Part model, mm, in its own coordinate system. Face numbers are marked on the shaded views. A direction names the side the tool comes from. Give positions to 0.01 mm unless a question says otherwise; leave off trailing zeros. Write each loop counter-clockwise with the first axis right and the second up, starting at its lowest first coordinate (ties: lowest second). Pieces come first, ordered by that corner, then holes.
```python
from build123d import *

# Parameters (mm, degrees)
SKETCH1_R           = 10
BOSS_EXTRUDE1_DEPTH = 8
BOSS_EXTRUDE2_DEPTH = 15
SKETCH3_R           = 5
CUT_EXTRUDE1_DEPTH  = 23.5


with BuildPart() as part:
    # Sketch1 → Boss-Extrude1 (new body)
    with BuildSketch(Plane.XY):
        with BuildLine():
            Line((12.990381057, 7.5), (32.990381057, 7.5))
            Line((32.990381057, 7.5), (32.990381057, -7.5))
            Line((32.990381057, -7.5), (12.990381057, -7.5))
            ThreePointArc((12.990381057, -7.5), (-15, 0), (12.990381057, 7.5))
        make_face()
        Circle(SKETCH1_R, mode=Mode.SUBTRACT)
    extrude(amount=BOSS_EXTRUDE1_DEPTH)

    # Sketch2 → Boss-Extrude2 (add)
    with BuildSketch(Plane(origin=(0, 7.5, 0), x_dir=(1, 0, 0), z_dir=(0, 1, 0))):
        with BuildLine():
            ThreePointArc((21.676672558, -8), (44.990381057, -4), (21.676672558, 0))
            Line((21.676672558, 0), (32.990381057, 0))
            Line((32.990381057, 0), (32.990381057, -8))
            Line((32.990381057, -8), (21.676672558, -8))
        make_face()
    extrude(amount=-BOSS_EXTRUDE2_DEPTH)

    # Sketch3 → Cut-Extrude1 (cut, through all)
    with BuildSketch(Plane(origin=(0, 7.5, 0), x_dir=(1, 0, 0), z_dir=(0, 1, 0))):
        with Locations((32.990381057, -4)):
            Circle(SKETCH3_R)
    extrude(amount=-CUT_EXTRUDE1_DEPTH, mode=Mode.SUBTRACT)


solid = part.part
```
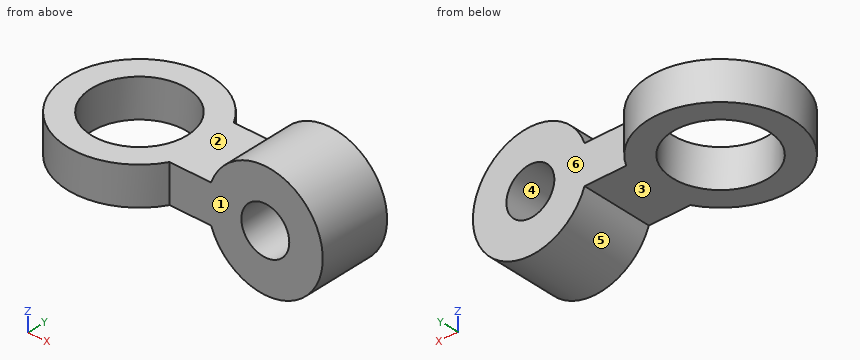
1) Saw through at A-A, the plane y = 0. Write the cut outline in (x, z), then the cut area to 3 significant figures.
Answers follow:
outline: (-15, 0) - (-10, 0) - (-10, 8) - (-15, 8) - close; (10, 0) - (21.68, 0) arc R12 ccw (long way) to (21.68, 8) - (10, 8) - close; hole circle Ø10 at (32.99, 4)
area: 504 mm2
2) Pin check, flat tips, straight feed: pin 1 Ø5 at (y, z) = (6.5, -4.5) entering from -X; pin 2 Ø5 at (x, y) = (39, -3) entering from +Z; pin 3 Ø3 at (y, z) = (-6, -4) entering from +X; pin 4 Ø3 at (y, z) = (1, 5) entering from +X. Stop position of each tip, or through.
Answers follow:
pin 1: stops at x = 22.6
pin 2: stops at z = 15.48
pin 3: stops at x = 43.08
pin 4: stops at x = 44.99
3) Wall check: L1, parallel to X at y = 0.5, z = 4; L2, parallel to X at y = -4, z = 4; L3, parallel to Z at x = -8, y = -10. Give the ranges that are in metal, low to high.
Answers follow:
L1: x = -14.99 to -9.99, 9.99 to 27.99, 37.99 to 44.99
L2: x = -14.46 to -9.17, 9.17 to 27.99, 37.99 to 44.99
L3: z = 0 to 8
4) Two-plate mould, pull along X, no slides. Class the marked faces 4, 5 and 6: +X half, -X half, draft (parallel to the pull), parting line (faces both ways), or undercut.
Answers follow:
face 4: undercut
face 5: parting line
face 6: draft
5) Saw through at B-B, the plane z = 1. Write the cut outline in (x, y), then the cut area to 3 significant figures.
Answers follow:
outline: (12.99, -7.5) - (28.99, -7.5) - (28.99, 7.5) - (12.99, 7.5) arc R15 ccw (long way) to start; (36.99, -7.5) - (44.61, -7.5) - (44.61, 7.5) - (36.99, 7.5) - close; hole circle Ø20 at (0, 0)
area: 727 mm2
6) Saw through at C-C, the plane x = 0. Write the cut outline in (y, z), then the cut area to 3 significant figures.
Answers follow:
outline: (-15, 0) - (-10, 0) - (-10, 8) - (-15, 8) - close; (10, 0) - (15, 0) - (15, 8) - (10, 8) - close
area: 80.0 mm2
7) 3-axis set-ups, long thin cutter, end or side, ignore diameter. For the marked faces 1, 2 and 3: which of +Z, -Z, +X, -X, +Y, -Y reach the whole face in a straight line?
Answers follow:
face 1: +Z, -Z, +X, -Y
face 2: +Z, -X, +Y, -Y
face 3: -Z, -X, +Y, -Y
8) Saw through at D-D, the plane x = 14. Write the cut outline in (y, z), then the cut area to 3 significant figures.
Answers follow:
outline: (-7.5, 0) - (7.5, 0) - (7.5, 8) - (-7.5, 8) - close
area: 120 mm2
